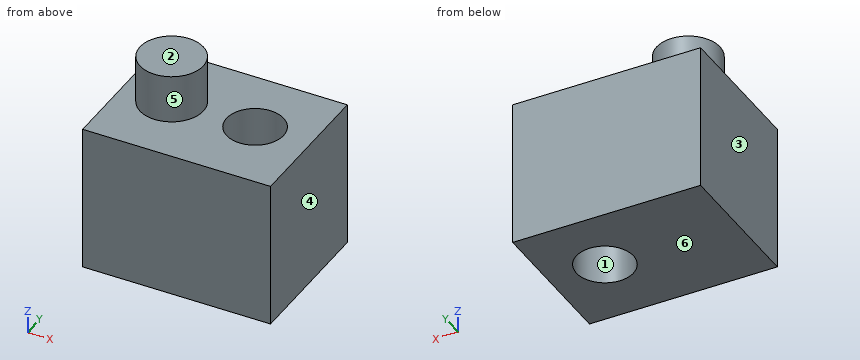
from build123d import *

# Parameters (mm, degrees)
F0_W     = 98.734826
F0_H     = 75.453311
F1_DEPTH = 77.475334
F2_R     = 14.996308
F3_DEPTH = 122.458426
F4_R     = 16.637872
F5_DEPTH = 25.4


with BuildPart() as f1:
    # F0 (on Top) → F1 (new body)
    with BuildSketch(Plane.XY):
        with Locations((6.044999, -1.713828)):
            Rectangle(F0_W, F0_H)
    extrude(amount=F1_DEPTH)

    # F2 (on face) → F3 (cut)
    with BuildSketch(Plane.XY.offset(77.475334)):
        with Locations((26.188662, 0)):
            Circle(F2_R)
    extrude(amount=-F3_DEPTH, mode=Mode.SUBTRACT)

    # F4 (on face) → F5 (join)
    with BuildSketch(Plane.XY.offset(77.475334)):
        with Locations((-17.651428, 0)):
            Circle(F4_R)
    extrude(amount=F5_DEPTH)


solid = f1.part
Source: CAD feature listing. Evaluate the final solid. Frame: model axes, mm. Face numbers are marked on the shaded views. A direction names the side the tool comes from. Give positions to 0.01 mm unless a question says otherwise; leave off trailing zeros. Write each loop counter-clockwise with the first axis right and the second up, starting at its lowest first coordinate (ties: lowest second). Pieces come first, ordered by that corner, then holes. Notation, with made-up numbers: M 86.5,83 L 103.5,83 A15 ccw 103.5,96 Z; hole C 70,84 d5. An arc over 180 degrees is marked long. Return JSON: item names as keys, results as strings. Group by question number.
1) Pull-direction query (X, two-part tool) for the marked faces 1, 2, 3 and 4; classes: pulls with the +X half, pulls with the -X half, needs draft (parallel to the pull), parting line crosses it, or undercut.
2) Cut plane D-D, the plane x = -26. Output: boundary loops of the cut face in (y, z), plus the area to 3 significant figures.
3) Cut plane B-B, the plane y = 4.5. Output: boundary loops of the cut face in (x, z).
4) Pin query (flat end, axial travel): P1, Ø12, axis at y = 15.5, z = 89, coming from the -X side; P2, Ø1.5, axis at y = 1.5, z = 78.5, coming from the +X side; P3, Ø8, axis at x = 37, y = -5.5, coming from the +Z side; P4, Ø24, axis at x = 26.19, y = 0, coming from the -Z side (3 decimals). Return the tip coordinate at first contact, or that it passes through.
5) Material intervals for line 1 along Z through (x, y) = (9, 17); line 2 along Y through (x, z) = (16.5, 39.5); line 3 along X through (y, z) = (3, 61), sorted ascending. Write a range as [from, to].
6) Set-up query: the marked faces 5 and 6. Return all of +Z, -Z, +X, -X, +Y, -Y with unobstructed straight access to the full face (end or side cutting, diameter ignored); none if empty.
7) Cut plane A-A, the plane z = 9.5. Output: boundary loops of the cut face in (x, y), plus the area to 3 significant figures.
8) Cut plane C-C, the plane x = 31.5. Output: boundary loops of the cut face in (y, z), plus the area to 3 significant figures.
Recorded:
{
 "1": {"face 1": "undercut", "face 2": "needs draft", "face 3": "pulls with the -X half", "face 4": "pulls with the +X half"},
 "2": {"outline": "M -39.44,0 L 36.01,0 L 36.01,77.48 L 14.39,77.48 L 14.39,102.88 L -14.39,102.88 L -14.39,77.48 L -39.44,77.48 Z", "area": "6,580 mm²"},
 "3": {"outline": "M -43.32,0 L 11.88,0 L 11.88,77.48 L -1.63,77.48 L -1.63,102.88 L -33.67,102.88 L -33.67,77.48 L -43.32,77.48 Z; M 40.49,0 L 55.41,0 L 55.41,77.48 L 40.49,77.48 Z"},
 "4": {"P1": "stops at x = -31.31", "P2": "stops at x = -1.03", "P3": "stops at z = 77.48", "P4": "passes through"},
 "5": {"line 1": "z = [0, 77.48]", "line 2": "y = [-39.44, -11.45], [11.45, 36.01]", "line 3": "x = [-43.32, 11.5], [40.88, 55.41]"},
 "6": {"face 5": "+Z", "face 6": "-Z, +X, -X, +Y, -Y"},
 "7": {"outline": "M -43.32,-39.44 L 55.41,-39.44 L 55.41,36.01 L -43.32,36.01 Z; hole C 26.19,0 d29.99", "area": "6,740 mm²"},
 "8": {"outline": "M -39.44,0 L -14.02,0 L -14.02,77.48 L -39.44,77.48 Z; M 14.02,0 L 36.01,0 L 36.01,77.48 L 14.02,77.48 Z", "area": "3,670 mm²"}
}
